Source: three-view drawing plus pictorial views. Frame: mm from the lowest corner of the part. Give positions to 0.01 mm unless a question says otherwise; leave off trailing zeros. Write each loop counter-clockwise with the first axis right and the second up, starting at its lowest first coordinate (ties: lowest second). Pieces come first, ordered by that corner, then holes.
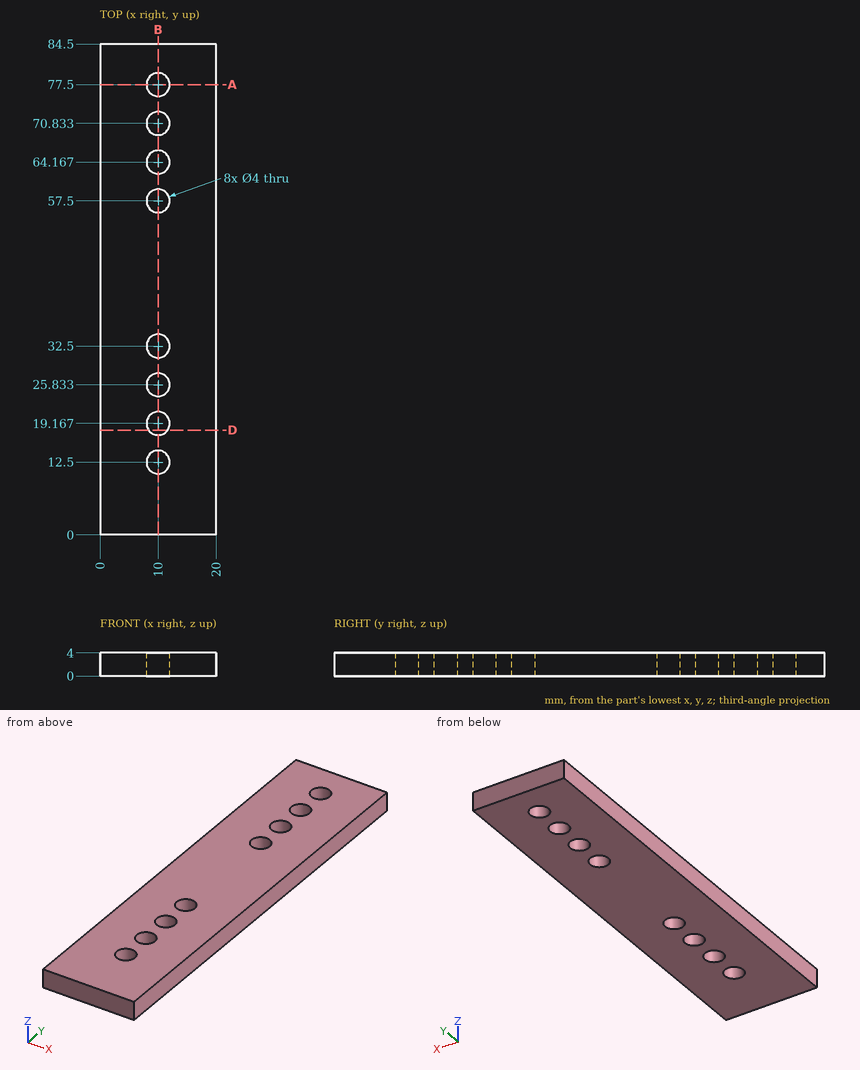
Q1. Section D-D on y = 18. Output: boundary loops of the cut face in (x, z) (1 decimal).
Filled sheet:
outline: (0, 0) - (8.4, 0) - (8.4, 4) - (0, 4) - close; (11.6, 0) - (20, 0) - (20, 4) - (11.6, 4) - close
Q2. Ray query, line 1 along X through (y, z) = (78, 0.2); line 2 along X through (y, z) = (25.5, 0.9). Return the intervals inside material, ascending.
Filled sheet:
line 1: x = 0 to 8.06, 11.94 to 20
line 2: x = 0 to 8.03, 11.97 to 20
Q3. Section A-A on y = 77.5. Output: boundary loops of the cut face in (x, z).
Filled sheet:
outline: (0, 0) - (8, 0) - (8, 4) - (0, 4) - close; (12, 0) - (20, 0) - (20, 4) - (12, 4) - close
Q4. Pin query (flat end, axial travel): P1, Ø3, axis at x = 10, y = 25.83, coming from the -Z side. Return the tip coordinate at first contact, or that it passes through.
Filled sheet:
P1: passes through
Q5. Section B-B on x = 10. Count the separate pieces of the cut face and the enclosed holes in it, plus the area to 3 significant figures.
Filled sheet:
separate pieces: 9
enclosed holes: 0
area: 210 mm2
